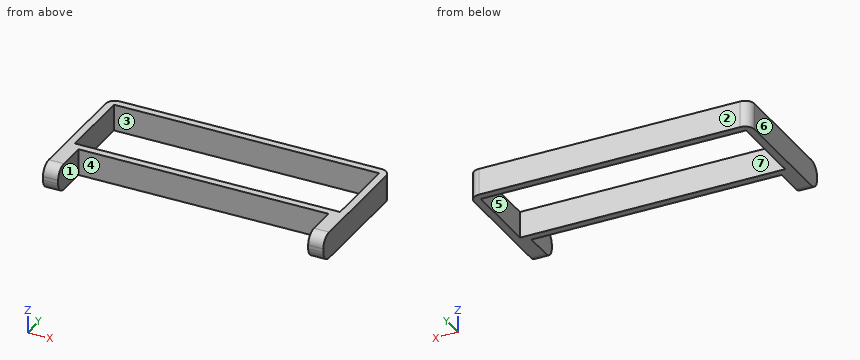
from build123d import *

# Parameters (mm, degrees)
SKETCH_W    = 140
SKETCH_H    = 40.5
PAD_DEPTH   = 14
FILLET_R    = 6
FILLET001_R = 6
FILLET002_R = 5


with BuildPart() as part:
    # Sketch → Pad (new body)
    with BuildSketch(Plane.XY):
        Polygon((-4, 44.5), (144, 44.5), (144, -25), (136, -25), (136, -4), (4, -4), (4, -25), (-4, -25), align=None)
        with Locations((70, 20.25)):
            Rectangle(SKETCH_W, SKETCH_H, mode=Mode.SUBTRACT)
    extrude(amount=PAD_DEPTH)

    # Fillet
    fillet_edges = [part.edges().sort_by_distance(p)[0] for p in [
        (0, -25, 14),
        (0, -25, 0),
    ]]
    fillet(fillet_edges, radius=FILLET_R)

    # Fillet001
    fillet001_edges = [part.edges().sort_by_distance(p)[0] for p in [
        (140, -25, 0),
        (140, -25, 14),
    ]]
    fillet(fillet001_edges, radius=FILLET001_R)

    # Fillet002
    fillet002_edges = [part.edges().sort_by_distance(p)[0] for p in [
        (-4, 44.5, 7),
        (144, 44.5, 7),
    ]]
    fillet(fillet002_edges, radius=FILLET002_R)


solid = part.part
Build history of the part. All positions in model axes, mm. Face numbers are marked on the shaded views. A direction names the side the tool comes from. Give positions to 0.01 mm unless a question says otherwise; leave off trailing zeros. Order: outer loops, then holes, each group sorted by start corner. A loop starts at its lowest first (then second) coordinate and runs counter-clockwise, first axis right, second up. Notation, with made-up numbers: M -39.75,-2.5 L -26.75,-2.5 A10 ccw -26.75,13.5 Z; hole C 74.5,62 d4. An arc over 180 degrees is marked long. Put each result on its own line as item: value.
Item 1: Probe line 1 (X direction, y = 22, z = 10); line 2 (Y direction, x = 60, z = 3.25); line 3 (X direction, y = -11.5, z = 6.5). List the from-to ranges inside material, lowest first. Write a range as [from, to].
From the geometry:
line 1: x = [-4, 0], [140, 144]
line 2: y = [-4, 0], [40.5, 44.5]
line 3: x = [-4, 4], [136, 144]
Item 2: Slice it at B-B, the plane y = 36.5. Write the cut outline in (x, z), plus the area to 3 significant figures.
From the geometry:
outline: M -4,0 L 0,0 L 0,14 L -4,14 Z; M 140,0 L 144,0 L 144,14 L 140,14 Z
area: 112 mm2
Item 3: Flat gauge pin, fed straight in: pin 1 Ø2 at (x, z) = (73.5, 12) entering from -Y. Where does the tip first touch, or does it go through?
From the geometry:
pin 1: stops at y = -4
Item 4: Slice it at A-A, the plane x = 86. Write the cut outline in (y, z), plus the area to 3 significant figures.
From the geometry:
outline: M -4,0 L 0,0 L 0,14 L -4,14 Z; M 40.5,0 L 44.5,0 L 44.5,14 L 40.5,14 Z
area: 112 mm2
Item 5: Slice it at C-C, the plane z = 10.5. Write the cut outline in (x, y).
From the geometry:
outline: M -4,-24.45 L 4,-24.45 L 4,-4 L 136,-4 L 136,-24.45 L 144,-24.45 L 144,39.5 A5 ccw 139,44.5 L 1,44.5 A5 ccw -4,39.5 Z; hole M 0,0 L 140,0 L 140,40.5 L 0,40.5 Z
Item 6: Two-plate mould, pull along Y, no slides. Class the marked faces 4, 5, 6 and 7: +Y half, -Y half, draft (parallel to the pull), parting line (faces both ways), or undercut.
From the geometry:
face 4: -Y half
face 5: undercut
face 6: draft
face 7: undercut
Item 7: 3-axis set-ups, long thin cutter, end or side, ignore diameter. For the marked faces 1, 2 and 3: which of +Z, -Z, +X, -X, +Y, -Y reach the whole face in a straight line?
From the geometry:
face 1: +Z, -Z, -Y
face 2: +Z, -Z, +X, -X, +Y
face 3: +Z, -Z
